Answer from the drawing. Dimensions are ordinates in mm from the lowest x, y and z of the part. A direction names the side the tool comes from. Give positions to 0.01 mm unless a question says otherwise; leave off trailing zeros. Write each loop counter-clockwise with the first axis right and the second up, starting at its lowest first coordinate (ties: lowest second). Pieces come first, ordered by that corner, then holes. Notation, with made-up numbers: (-38, -29) -> (14, -29) arc R29 ccw to (14, -4) -> close; hole circle Ø5 at (17.5, 36). An arc over 180 degrees is marked (long way). Use a Markdown table: item, result. Add a question column.
Q1. Section A-A, the plane x = 36 is taken. Give the vertices of the cut face in (y, z), plus the area to 4 significant figures.
Q2. Each of these flat-tipped pins is pushed along its axis until it touches: pin 1 Ø6 at (x, y) = (80, 62) entering from +Z (1 decimal); pin 2 Ø1.5 at (y, z) = (10, 50.5) entering from -X; pin 3 Ø1 at (x, y) = (68, 54.5) entering from -Z. Where does it stop, or does it pass through?
Q3. Section B-B, the plane z = 38 is taken. Give the vertices of the cut face in (x, y), plus the area to 3 significant figures.
Q4. Section C-C, the plane y = 66.5 is taken. Give the vertices of the cut face in (x, z) (3 decimals), plus the area to 3 significant figures.
Q5. Section D-D, the plane x = 16 is taken. Give the vertices of the cut face in (y, z), plus the area to 3 significant figures.
Q6. Consider line 1 (Y direction, x = 47, z = 7.5); line 2 (X direction, y = 34, z = 48.5); line 3 (Y direction, x = 73.5, z = 12). Determine where each line is inside the solid, lowest interval first.
Q7. For the marked faces 1 and 2, determine the directions among +Z, -Z, +X, -X, +Y, -Y from which every point of the face is accessible in a straight line to the end or side of a thin tool.
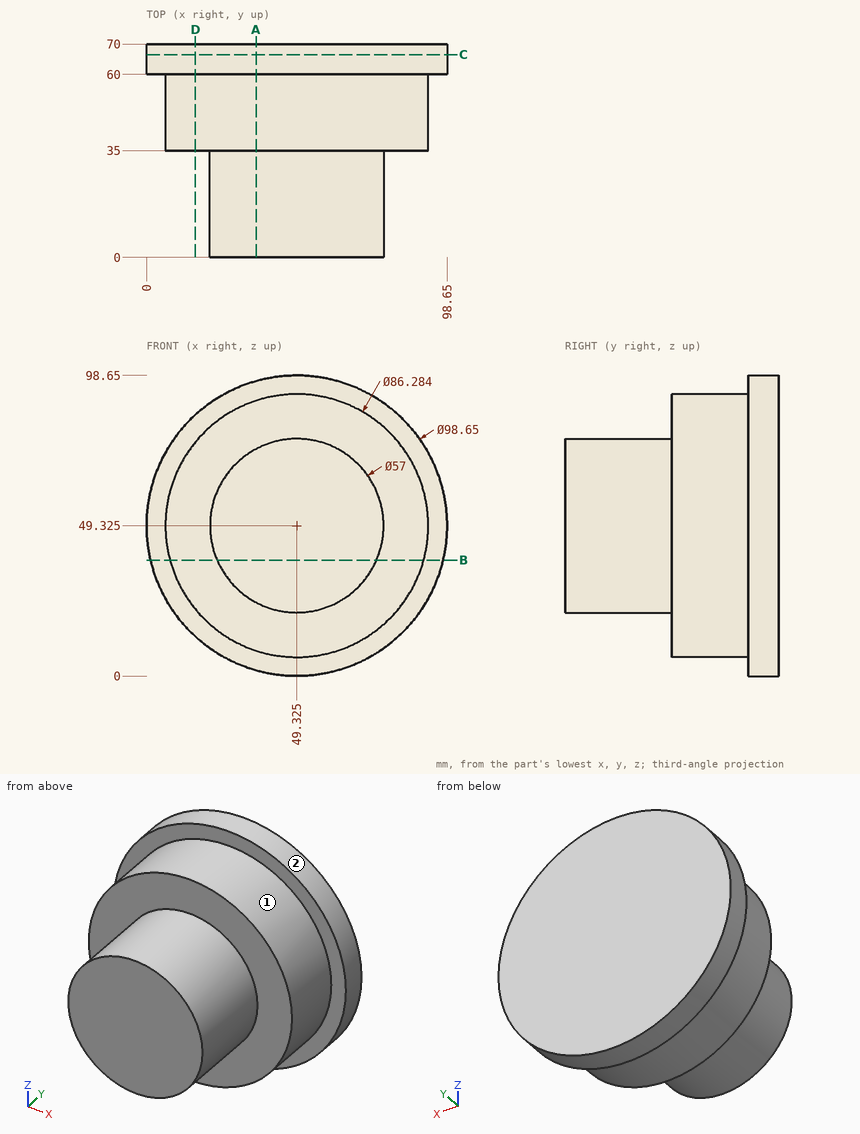
Result set:
| question | item | result |
|---|---|---|
| 1 | outline | (0, 24.13) -> (35, 24.13) -> (35, 8.29) -> (60, 8.29) -> (60, 1.83) -> (70, 1.83) -> (70, 96.82) -> (60, 96.82) -> (60, 90.36) -> (35, 90.36) -> (35, 74.52) -> (0, 74.52) -> close |
| 1 | area | 4,765 mm2 |
| 2 | pin 1 | stops at z = 90.2 |
| 2 | pin 2 | stops at x = 20.83 |
| 2 | pin 3 | stops at z = 10.2 |
| 3 | outline | (1.32, 60) -> (7.7, 60) -> (7.7, 35) -> (23.17, 35) -> (23.17, 0) -> (75.48, 0) -> (75.48, 35) -> (90.95, 35) -> (90.95, 60) -> (97.33, 60) -> (97.33, 70) -> (1.32, 70) -> close |
| 3 | area | 4,870 mm2 |
| 4 | outline | circle Ø98.65 at (49.325, 49.325) |
| 4 | area | 7,640 mm2 |
| 5 | outline | (35, 21.93) -> (60, 21.93) -> (60, 12.96) -> (70, 12.96) -> (70, 85.69) -> (60, 85.69) -> (60, 76.72) -> (35, 76.72) -> close |
| 5 | area | 2,100 mm2 |
| 6 | line 1 | y = 35 to 70 |
| 6 | line 2 | x = 20.84 to 77.81 |
| 6 | line 3 | y = 60 to 70 |
| 7 | face 1 | -Y |
| 7 | face 2 | +Y, -Y |
